Could you check a few things on this model? Use its own coordinates, in mm. Round coordinates to 2 decimals unless told otherwise and drop trailing zeros. Order: outer loops, then holes, each group sorted by start corner. A loop starts at its lowest first (then second) coordinate and runs counter-clockwise, first axis right, second up. Notation, with made-up numbers: (43.25, 6) -> (86.25, 6) arc R32 ccw to (86.25, 42) -> close; hole circle Ø6 at (35.5, -38.75). An arc over 180 degrees is marked (long way). One line per question, with ' | ' between items.
```python
from build123d import *

# Parameters (mm, degrees)
SCHIZZO1_R                   = 1.5
ESTRUSIONE_ESTRUSIONE1_DEPTH = 4
SCHIZZO2_R                   = 1.5
TAGLIO_ESTRUSIONE1_DEPTH     = 10


with BuildPart() as part:
    # Schizzo1 → Estrusione-Estrusione1 (new body)
    with BuildSketch(Plane.XY):
        with BuildLine():
            ThreePointArc((-1.538071066, 7.340595166), (-7.378454008, -1.344773756), (1.150548918, -7.411223731))
            ThreePointArc((1.150548918, -7.411223731), (75.443261143, -2.885528453), (149.288277512, -12.20231786))
            ThreePointArc((149.288277512, -12.20231786), (152.810661847, -12.473685396), (156.268292683, -11.748688334))
            ThreePointArc((156.268292683, -11.748688334), (178.283063002, -6.762377854), (200.846153846, -7.410711103))
            ThreePointArc((200.846153846, -7.410711103), (209.378154672, -1.346415107), (203.538071066, 7.340595166))
            ThreePointArc((203.538071066, 7.340595166), (101, 17.967584078), (-1.538071066, 7.340595166))
        make_face()
        Circle(SCHIZZO1_R, mode=Mode.SUBTRACT)
        with Locations((202, 0)):
            Circle(SCHIZZO1_R, mode=Mode.SUBTRACT)
        with Locations((152, 0)):
            Circle(SCHIZZO1_R, mode=Mode.SUBTRACT)
    extrude(amount=ESTRUSIONE_ESTRUSIONE1_DEPTH)

    # Schizzo2 → Taglio-Estrusione1 (cut)
    with BuildSketch(Plane.XY.offset(4)):
        with Locations((21.792647349, 3.923925867)):
            Circle(SCHIZZO2_R)
        with Locations((115.643522851, 5.673925867)):
            Circle(SCHIZZO2_R)
        with Locations((180.602574062, 1.58663817)):
            Circle(SCHIZZO2_R)
    extrude(amount=-TAGLIO_ESTRUSIONE1_DEPTH, mode=Mode.SUBTRACT)


solid = part.part
```
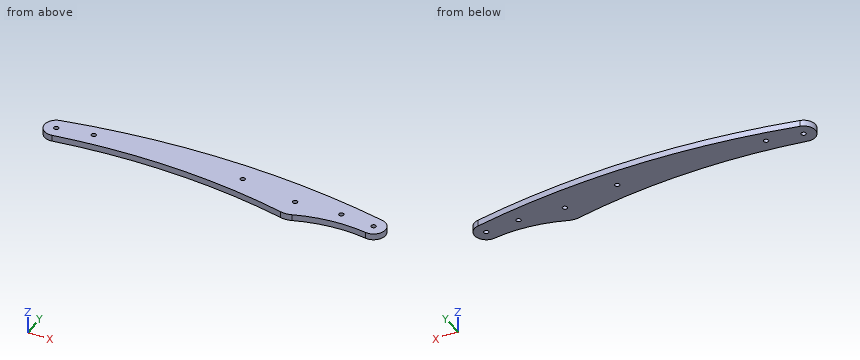
1. I need wall thicknesses on probe 1 along X at (y, z) = (5, 0.55); probe 2 along X at (y, z) = (1, 1.65); probe 3 along Y at (x, z) = (71.5, 1.4). Which ranges of each line are inside material? Lowest first, please.
From the geometry:
probe 1: x = -5.59 to 20.75, 22.84 to 114.3, 116.98 to 207.59 | probe 2: x = -7.43 to -1.12, 1.12 to 150.88, 153.12 to 179.22, 181.98 to 200.88, 203.12 to 209.43 | probe 3: y = -2.78 to 17.1
2. I'm going to push flat-ended pins straight in: pin 1 (12 mm diameter, centred on x = 114.5, y = 10.5, fed in from -Z); pin 2 (1.5 mm diameter, centred on y = 1, z = 3, fed in from -X). Where does each tip first touch, or does it pass through?
From the geometry:
pin 1: stops at z = 0 | pin 2: stops at x = -7.5
3. I want a section at A-A on z = 1.1. List the corners of the cut face in (x, y) for me.
From the geometry:
outline: (-1.54, 7.34) arc R7.5 ccw to (1.15, -7.41) arc R400 cw to (149.29, -12.2) arc R12.5 ccw to (156.27, -11.75) arc R90 cw to (200.85, -7.41) arc R7.5 ccw to (203.54, 7.34) arc R500 ccw to start; hole circle Ø3 at (0, 0); hole circle Ø3 at (21.79, 3.92); hole circle Ø3 at (115.64, 5.67); hole circle Ø3 at (152, 0); hole circle Ø3 at (180.6, 1.59); hole circle Ø3 at (202, 0)
4. I want a section at B-B on x = 189.5. List the corners of the cut face in (y, z) for me, and give its area (3 significant figures).
From the geometry:
outline: (-6.37, 0) -> (10.07, 0) -> (10.07, 4) -> (-6.37, 4) -> close | area: 65.8 mm²
